from build123d import *

# Parameters (mm, degrees)
F0_W     = 584.2
F0_H     = 219.71
F1_DEPTH = 5.334
F2_W     = 571.5
F2_H     = 213.36
F2_W_2   = 546.1
F2_H_2   = 187.96
F3_DEPTH = 12.7
F4_R     = 25.4
F6_DEPTH = 12.7
F8_DEPTH = 5.334


# Not quite as in the source:
# - a feature names something its author has since deleted; it is built from what else it names


with BuildPart() as f1:
    # F0 (on Front) → F1 (new body)
    with BuildSketch(Plane.XZ):
        with Locations((-292.1, 109.855)):
            Rectangle(F0_W, F0_H)
    extrude(amount=F1_DEPTH)

    # F2 (on face) → F3 (join)
    with BuildSketch(Plane.XZ.offset(5.334)):
        with Locations((-292.1, 113.03)):
            Rectangle(F2_W, F2_H)
        with Locations((-292.1, 113.03)):
            Rectangle(F2_W_2, F2_H_2, mode=Mode.SUBTRACT)
    extrude(amount=F3_DEPTH)

    # F4
    f4_edges = [f1.edges().sort_by_distance(p)[0] for p in [
        (-565.15, -11.684, 207.01),
        (-19.05, -11.684, 207.01),
        (-19.05, -11.684, 19.05),
        (-565.15, -11.684, 19.05),
    ]]
    fillet(f4_edges, radius=F4_R)

    # F5 (on face) → F6 (cut)
    with BuildSketch(Plane.XZ.offset(18.034)):
        Polygon((-118.11, 219.71), (-125.73, 207.01), (-118.11, 207.01), (-113.5820166854, 214.5566388576), (-110.49, 219.71), align=None)
        Polygon((-56.5979833146, 214.5566388576), (-52.07, 207.01), (-44.45, 207.01), (-52.07, 219.71), (-59.69, 219.71), align=None)
        Polygon((-59.69, 219.71), (-110.49, 219.71), (-113.5820166854, 214.5566388576), (-56.5979833146, 214.5566388576), align=None)
    extrude(amount=-F6_DEPTH, mode=Mode.SUBTRACT)

    # F7 (on face) → F8 (join)
    with BuildSketch(Plane(origin=(0, 0, 0), x_dir=(-1, 0, 0), z_dir=(0, 1, 0))):
        with BuildLine():
            Line((-5.08, 229.87), (0, 176.1275827885))
            Line((0, 176.1275827885), (0, 219.71))
            Line((0, 219.71), (148.0852009026, 219.71))
            add(Edge.make_bspline(
                [(148.0852009026, 219.71), (115.3779899576, 221.1840971885), (80.5489949788, 225.5270485943), (45.72, 229.87)],
                knots=[0.812101374, 0.812101374, 0.812101374, 0.812101374, 1, 1, 1, 1], degree=3))
            Line((45.72, 229.87), (-5.08, 229.87))
        make_face()
        with BuildLine():
            add(Edge.make_bspline(
                [(393.7, 219.71), (356.8171998762, 221.731425099), (324.4585999381, 229.87), (292.1, 229.87)],
                knots=[0.2719218593, 0.2719218593, 0.2719218593, 0.2719218593, 0.5, 0.5, 0.5, 0.5], degree=3))
            add(Edge.make_bspline(
                [(292.1, 229.87), (259.7414000619, 229.87), (227.3828001238, 221.731425099), (190.5, 219.71)],
                knots=[0.5, 0.5, 0.5, 0.5, 0.7280781407, 0.7280781407, 0.7280781407, 0.7280781407], degree=3))
            Line((190.5, 219.71), (393.7, 219.71))
        make_face()
        Polygon((584.2, 183.2547038794), (584.2, 0), (589.28, 0), align=None)
        with BuildLine():
            Line((584.2, 219.71), (584.2, 183.2547038794))
            Line((584.2, 183.2547038794), (589.28, 229.87))
            Line((589.28, 229.87), (538.48, 229.87))
            add(Edge.make_bspline(
                [(538.48, 229.87), (503.6510050212, 225.5270485943), (468.8220100424, 221.1840971885), (436.1147990974, 219.71)],
                knots=[0, 0, 0, 0, 0.187898626, 0.187898626, 0.187898626, 0.187898626], degree=3))
            Line((436.1147990974, 219.71), (584.2, 219.71))
        make_face()
        Polygon((-5.08, 0), (0, 0), (0, 176.1275827885), align=None)
    extrude(amount=-F8_DEPTH)


solid = f1.part
Could you check a few things on this model? Use its own coordinates, in mm. A direction names the side the tool comes from. Coordinates: 2 decimals unless noted, no trailing zeros. Order: outer loops, then holes, each group sorted by start corner. A loop starts at its lowest first (then second) coordinate and runs counter-clockwise, first axis right, second up.
Q1. Please list where these lines run through material, in increasing order: L1, parallel to Z at x = -413.5, y = -16.25; L2, parallel to Z at x = -102, y = -17; L3, parallel to X at y = -8.75, z = 158.
Q2. Which directions (+Z, -Z, +X, -X, +Y, -Y) give clear straight access to the entire face, cutting with the end or side of a thin tool? Please do faces 1 (the flat face through (-292, -5.334, 224)), 2 (the flat face through (-577.85, -12, 112)), 3 (the flat face through (-19.05, -12, 112)).
Q3. Will these pins go through, and if not, where does the flat tip stop? pin 1 (5 mm diameter, centred on y = -6.5, z = 29, fed in from +X); pin 2 (4 mm diameter, centred on x = -153.5, y = -14, fed in from +Z); pin 3 (12 mm diameter, centred on x = -371.5, z = 61.5, fed in from -Y).
Q4. Suppose I cut it at D-D on z = 125.5. Please give me the cut outline in (x, y).
Q5. Suppose I cut it at A-A on y = -10.25. Please give me the cut outline in (x, z), and give its area (3 significant figures).
Q6. Suppose I cut it at B-B on x = -400. Please give me the cut outline in (y, z).
Q7. Suppose I cut it at C-C on z = 77. Please give me the cut outline in (x, y), and give its area (3 significant figures).
Answer:
1. L1: z = 6.35 to 19.05, 207.01 to 219.71
1. L2: z = 6.35 to 19.05, 207.01 to 214.56
1. L3: x = -577.85 to -565.15, -19.05 to -6.35
2. face 1: +Z, +X, -X, -Y
2. face 2: +Z, -Z, -X, -Y
2. face 3: -Y
3. pin 1: stops at x = 4.31
3. pin 2: stops at z = 219.71
3. pin 3: stops at y = -5.33
4. outline: (-585.8, -5.33) - (-577.85, -5.33) - (-577.85, -18.03) - (-565.15, -18.03) - (-565.15, -5.33) - (-19.05, -5.33) - (-19.05, -18.03) - (-6.35, -18.03) - (-6.35, -5.33) - (1.46, -5.33) - (1.46, 0) - (-585.8, 0) - close
5. outline: (-577.85, 6.35) - (-6.35, 6.35) - (-6.35, 219.71) - (-52.07, 219.71) - (-44.45, 207.01) arc R25.4 cw to (-19.05, 181.61) - (-19.05, 44.45) arc R25.4 cw to (-44.45, 19.05) - (-539.75, 19.05) arc R25.4 cw to (-565.15, 44.45) - (-565.15, 181.61) arc R25.4 cw to (-539.75, 207.01) - (-125.73, 207.01) - (-118.11, 219.71) - (-577.85, 219.71) - close; (-118.11, 207.01) - (-52.07, 207.01) - (-56.6, 214.56) - (-113.58, 214.56) - close
5. area: 19,400 mm2
6. outline: (-18.03, 6.35) - (-5.33, 6.35) - (-5.33, 0) - (0, 0) - (0, 219.71) - (-18.03, 219.71) - (-18.03, 207.01) - (-5.33, 207.01) - (-5.33, 19.05) - (-18.03, 19.05) - close
7. outline: (-587.15, -5.33) - (-577.85, -5.33) - (-577.85, -18.03) - (-565.15, -18.03) - (-565.15, -5.33) - (-19.05, -5.33) - (-19.05, -18.03) - (-6.35, -18.03) - (-6.35, -5.33) - (2.86, -5.33) - (2.86, 0) - (-587.15, 0) - close
7. area: 3,470 mm2
